Geometry check sheet. Reference: the model listing, model coordinates, mm. Round coordinates to 2 decimals unless told otherwise and drop trailing zeros. Write each loop counter-clockwise with the first axis right and the second up, starting at its lowest first coordinate (ties: lowest second). Pieces come first, ordered by that corner, then holes. Notation, with made-up numbers: (19, 9) -> (48, 9) arc R32 ccw to (48, 36) -> close; hole circle Ø4 at (-28.75, 13). An arc over 180 degrees is marked (long way). Use a Markdown table: item, result.
```python
from build123d import *

# Parameters (mm, degrees)
F0_W     = 190.5
F0_H     = 3.175
F1_DEPTH = 9.525
F2_DEPTH = 12.7


with BuildPart() as f1:
    # F0 (on Right) → F1 (new body)
    with BuildSketch(Plane.YZ):
        with Locations((0, -68.2625)):
            Rectangle(F0_W, F0_H)
    extrude(amount=F1_DEPTH)

    # F0 (on Right) → F2 (join)
    with BuildSketch(Plane.YZ):
        Polygon((-95.25, -57.15), (-95.25, -66.675), (95.25, -66.675), (95.25, -57.15), (111.125, -57.15), (111.125, -44.45), (95.25, -44.45), (95.25, -31.75), (111.125, -31.75), (111.125, -19.05), (95.25, -19.05), (95.25, -6.35), (111.125, -6.35), (111.125, 6.35), (95.25, 6.35), (95.25, 19.05), (111.125, 19.05), (111.125, 31.75), (95.25, 31.75), (95.25, 44.45), (111.125, 44.45), (111.125, 57.15), (95.25, 57.15), (95.25, 69.85), (-95.25, 69.85), (-95.25, 57.15), (-111.125, 57.15), (-111.125, 44.45), (-95.25, 44.45), (-95.25, 31.75), (-111.125, 31.75), (-111.125, 19.05), (-95.25, 19.05), (-95.25, 6.35), (-111.125, 6.35), (-111.125, -6.35), (-95.25, -6.35), (-95.25, -19.05), (-111.125, -19.05), (-111.125, -31.75), (-95.25, -31.75), (-95.25, -44.45), (-111.125, -44.45), (-111.125, -57.15), align=None)
        with Locations((0, -71.4375)):
            Rectangle(F0_W, F0_H)
    extrude(amount=F2_DEPTH)


solid = f1.part
```
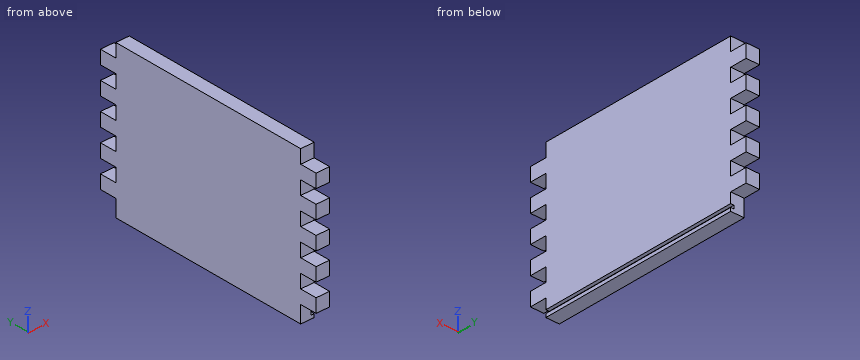
(1) Gauge pin test, flat ends, axial feed: pin 1 Ø4 at (x, y) = (8.5, 100.5) entering from -Z; pin 2 Ø4 at (x, z) = (8.5, 10.5) entering from -Y; pin 3 Ø6.5 at (x, y) = (9, 102.5) entering from +Z. Record the tip position at first contact, or that the pin passes through.
A:
| item | result |
|---|---|
| pin 1 | stops at z = -57.15 |
| pin 2 | stops at y = -95.25 |
| pin 3 | stops at z = 57.15 |
(2) Section check A-A on z = 13.5. Record the cut outline in (x, y).
A:
| item | result |
|---|---|
| outline | (0, -95.25) -> (12.7, -95.25) -> (12.7, 95.25) -> (0, 95.25) -> close |
(3) Thickness scan on line 1 (Z direction, x = 2.25, y = 100); line 2 (Z direction, x = 11, y = 74) (3 decimals). Record the ranges inside material, lowest first.
A:
| item | result |
|---|---|
| line 1 | z = -57.15 to -44.45, -31.75 to -19.05, -6.35 to 6.35, 19.05 to 31.75, 44.45 to 57.15 |
| line 2 | z = -73.025 to -69.85, -66.675 to 69.85 |
